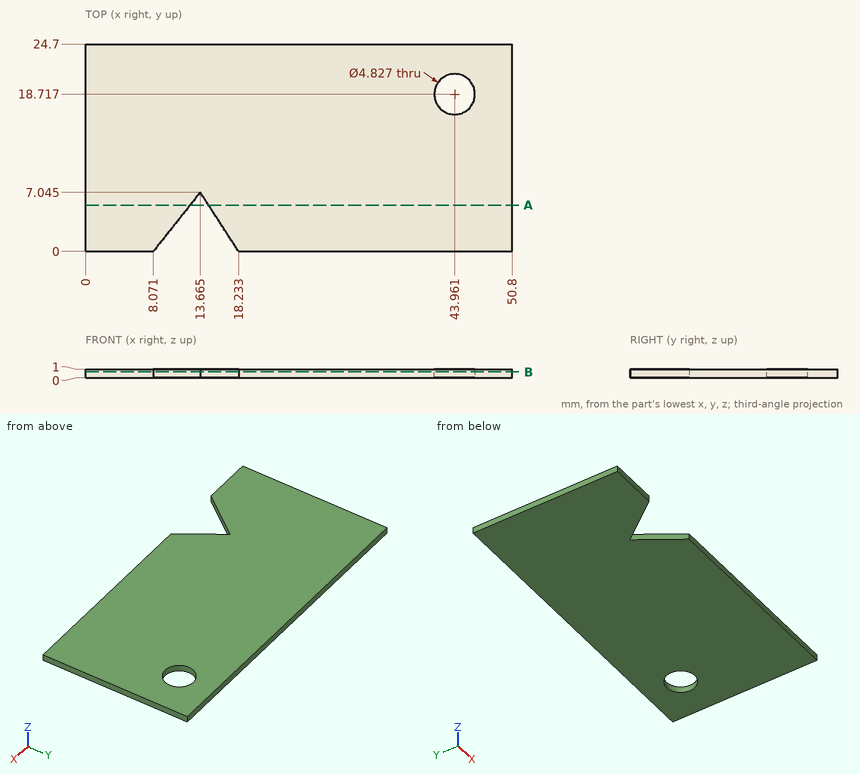
Geometry: see drawing. Coordinates: mm, zero at the bounding-box minimum. Coordinates: 2 decimals unless noted, no trailing zeros. Loops run counter-clockwise (first coordinate to the right, second up) from the corner with the lowest first, then second, coordinate; pieces in that order, holes last. Notation, with made-up numbers: M 45.25,33.5 L 56.25,33.5 A17 cw 56.25,50.5 Z; hole C -3.5,-34 d5. An arc over 180 degrees is marked long. Answer in a Markdown table with one row per item.
1. Section A-A, the plane y = 5.5. Output: boundary loops of the cut face in (x, z).
Response:
| item | result |
|---|---|
| outline | M 0,0 L 12.44,0 L 12.44,1 L 0,1 Z; M 14.67,0 L 50.8,0 L 50.8,1 L 14.67,1 Z |
2. Material intervals for line 1 (X direction, y = 19.5, z = 0.25); line 2 (X direction, y = 20.5, z = 0.35) (1 decimal); line 3 (Y direction, x = 44.5, z = 0.45) (1 decimal), sorted ascending.
Response:
| item | result |
|---|---|
| line 1 | x = 0 to 41.68, 46.24 to 50.8 |
| line 2 | x = 0 to 42.3, 45.6 to 50.8 |
| line 3 | y = 0 to 16.4, 21.1 to 24.7 |
3. First-contact query: pin 1 (3 mm diameter, centred on x = 43.96, y = 18.72, fed in from -Z). Flat tip, straight axial feed; report the tip coordinate or a pass-through.
Response:
| item | result |
|---|---|
| pin 1 | passes through |
4. Section B-B, the plane z = 0.7. Output: boundary loops of the cut face in (x, y) (1 decimal), then the cut area to 3 significant figures.
Response:
| item | result |
|---|---|
| outline | M 0,0 L 8.1,0 L 13.7,7 L 18.2,0 L 50.8,0 L 50.8,24.7 L 0,24.7 Z; hole C 44,18.7 d4.8 |
| area | 1,200 mm2 |
